Can you work these out from the model? Positions are in its coordinate system, mm. Coordinates: 2 decimals unless noted, no trailing zeros. Write each loop counter-clockwise with the first axis right and the second up, starting at its lowest first coordinate (ties: lowest second). Pieces come first, ordered by that corner, then holes. Notation, with made-up numbers: M -31,-9.5 L 24,-9.5 A26 cw 24,13.5 Z; hole C 25,3.25 d11. An arc over 180 degrees is marked long. Answer as a JSON object with one key per item and string values. Group by question number.
from build123d import *

# Parameters (mm, degrees)
BOSS_EXTRUDE1_DEPTH = 3.175


with BuildPart() as part:
    # Sketch1 → Boss-Extrude1 (new body)
    with BuildSketch(Plane(origin=(0, 0, 0), x_dir=(0, 0, -1), z_dir=(1, 0, 0))):
        with BuildLine():
            Line((0, 0), (9.525, 0))
            Line((9.525, 0), (38.322191876, 66.595518378))
            ThreePointArc((38.322191876, 66.595518378), (48.515936948, 74.170316159), (60.17277679, 69.129672857))
            Line((60.17277679, 69.129672857), (64.907025403, 62.758582188))
            ThreePointArc((64.907025403, 62.758582188), (64.579656991, 60.537514331), (66.800724848, 60.21014592))
            ThreePointArc((66.800724848, 60.21014592), (69.295454529, 64.381080761), (68.110198493, 69.094417346))
            Line((68.110198493, 69.094417346), (58.709682019, 81.745113939))
            ThreePointArc((58.709682019, 81.745113939), (51.186125331, 86.5864385), (42.337451795, 85.266095591))
            Line((42.337451795, 85.266095591), (0, 61.691247253))
            Line((0, 61.691247253), (0, 0))
        make_face()
    extrude(amount=BOSS_EXTRUDE1_DEPTH)


solid = part.part
Q1. We'd pull the mould along Y, two halves only. Please class faces 1 (the flat face through (3.175, 54, -26)), 2 (the cylindrical face through (1.565, 60.566, -64.559)), 3 (the flat face through (1.57, 32.83, -23.72)): pulls with the +Y half, pulls with the -Y half, needs draft (parallel to the pull), parting line crosses it, or undercut.
Q2. Will these pins go through, and if not, where does the flat tip stop? pin 1 (1 mm diameter, centred on x = 1, z = -54.5, fed in from +Y); pin 2 (1 mm diameter, centred on x = 2, z = -22, fed in from -Y).
Q3. If we section it at C-C on y = 15.5: List the corners of the cut face in (x, z) for me (1 decimal), and give its area (3 significant figures).
Q4. If we section it at B-B on z = -17: List the corners of the cut face in (x, y) for me (3 decimals).
Q5. Please list where these lines run through material, in increasing order: L1, parallel to Z at x = 1.8, y = 66.5; L2, parallel to Z at x = 2.15, y = 31.5; L3, parallel to Y at x = 2.3, z = -54.
Reply:
{
 "1": {"face 1": "needs draft", "face 2": "undercut", "face 3": "pulls with the -Y half"},
 "2": {"pin 1": "y = 85.63", "pin 2": "y = 27.69"},
 "3": {"outline": "M 0,-16.2 L 3.2,-16.2 L 3.2,0 L 0,0 Z", "area": "51.5 mm^2"},
 "4": {"outline": "M 0,17.286 L 3.175,17.286 L 3.175,71.157 L 0,71.157 Z"},
 "5": {"L1": "-69.25 to -62.13, -38.28 to -8.64", "L2": "-23.15 to 0", "L3": "73.6 to 85.63"}
}
